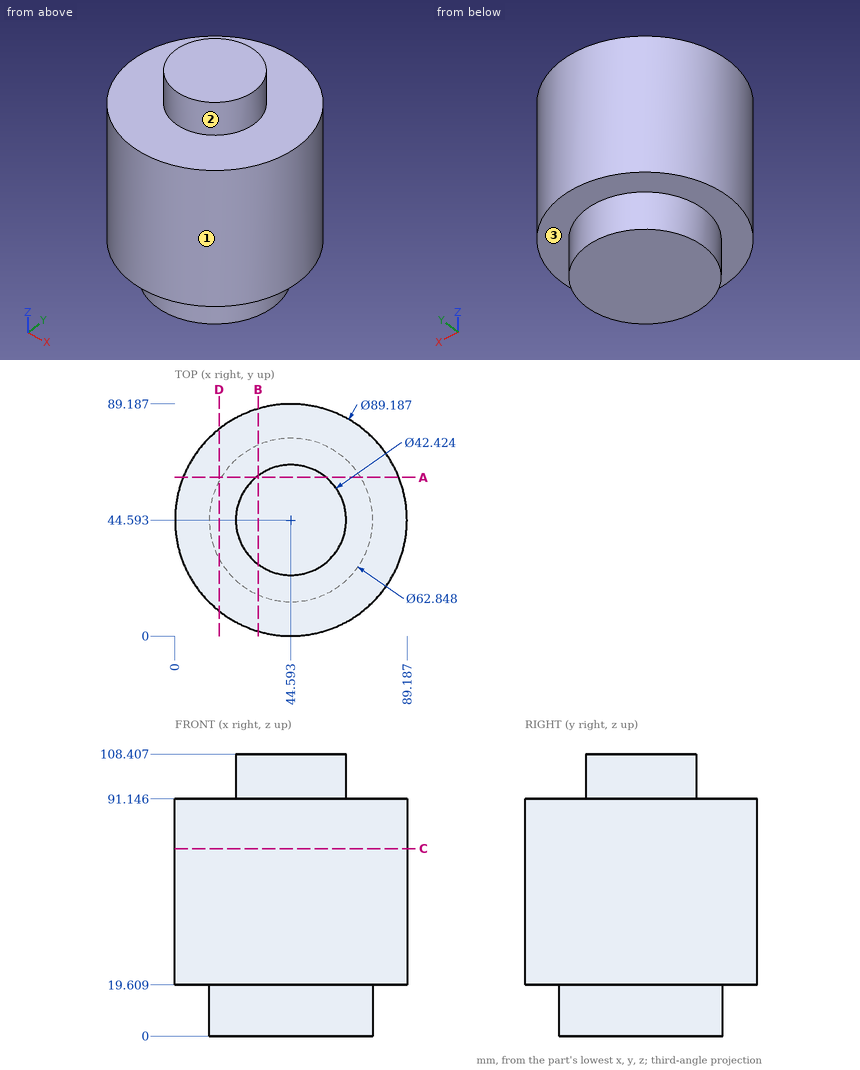
Input: dimensioned drawing with shaded views. Units: mm. Origin: part minimum x, y, z. A direction names the side the tool comes from. Round coordinates to 2 decimals unless told otherwise and drop trailing zeros. Order: outer loops, then holes, each group sorted by start corner. A loop starts at its lowest first (then second) coordinate and runs counter-clockwise, first axis right, second up.
1. Cut plane D-D, the plane x = 17. Output: boundary loops of the cut face in (y, z) (1 decimal), then the cut area to 3 significant figures.
The answers:
outline: (9.6, 19.6) - (29.6, 19.6) - (29.6, 0) - (59.6, 0) - (59.6, 19.6) - (79.6, 19.6) - (79.6, 91.1) - (9.6, 91.1) - close
area: 5,600 mm2
2. Set-up query: the marked faces 1, 2 and 3. Return all of +Z, -Z, +X, -X, +Y, -Y with unobstructed straight access to the full face (end or side cutting, diameter ignored); none if empty.
The answers:
face 1: +Z, -Z
face 2: +Z
face 3: -Z
3. Cut plane A-A, the plane y = 61. Output: boundary loops of the cut face in (x, z) (1 decimal).
The answers:
outline: (3.1, 19.6) - (17.8, 19.6) - (17.8, 0) - (71.4, 0) - (71.4, 19.6) - (86.1, 19.6) - (86.1, 91.1) - (58, 91.1) - (58, 108.4) - (31.1, 108.4) - (31.1, 91.1) - (3.1, 91.1) - close
4. Cut plane C-C, the plane z = 72. Output: boundary loops of the cut face in (x, y), then the cut area to 3 significant figures.
The answers:
outline: circle Ø89.19 at (44.59, 44.59)
area: 6,250 mm2
5. Cut plane B-B, the plane x = 32. Output: boundary loops of the cut face in (y, z) (1 decimal).
The answers:
outline: (1.8, 19.6) - (15.8, 19.6) - (15.8, 0) - (73.4, 0) - (73.4, 19.6) - (87.4, 19.6) - (87.4, 91.1) - (61.7, 91.1) - (61.7, 108.4) - (27.5, 108.4) - (27.5, 91.1) - (1.8, 91.1) - close
6. Material intervals for line 1 (Z direction, x = 69, y = 35.5); line 2 (Z direction, x = 19.5, y = 19); line 3 (X direction, y = 43.5, z = 10), sorted ascending.
The answers:
line 1: z = 0 to 91.15
line 2: z = 19.61 to 91.15
line 3: x = 13.19 to 76
7. Pin query (flat end, axial travel): P1, Ø1.5, axis at y = 71, z = 53, coming from the -X side; P2, Ø1.5, axis at y = 20.5, z = 74, coming from the -X side; P3, Ø4, axis at y = 32, z = 94, coming from the +X side. Return the tip coordinate at first contact, or that it passes through.
The answers:
P1: stops at x = 8.12
P2: stops at x = 6.6
P3: stops at x = 62.97
